Part model, mm, in its own coordinate system. A direction names the side the tool comes from. Round coordinates to 2 decimals unless told otherwise and drop trailing zeros. Loops run counter-clockwise (first coordinate to the right, second up) from the corner with the lowest first, then second, coordinate; pieces in that order, holes last.
(1) Mould opens along X. For faces 3 (the face through (516.086, -927, 1)), 4 (the face through (50, -1078, 1)), 5 (the face through (491, -1112.521, 1)) say: +X half, -X half, draft (parallel to the pull), parting line (faces both ways), or undercut.
(2) Flat gauge pins, fed straight in: pin 1 (5 mm diameter, centred on x = 457, z = 23, fed in from +Y); pin 2 (12 mm diameter, centred on x = 86.5, z = -0.5, fed in from +Y); pin 3 (2 mm diameter, centred on x = 250.5, z = 10, fed in from -Y). Where does each tip first touch, or does it go through?
(3) Cut at B-B on x = 88. List the corners of the cut face in (y, z), then the cut area to 3 significant figures.
(4) Cut at A-A on z = 4. List the corners of the cut face in (x, y), then the cut area to 3 significant figures.
(5) Tool access for faces 1 (the face through (255, -1042.521, 1)), 2 (the face through (0, -922, 1)): list every direction of +Z, -Z, +X, -X, +Y, -Y with a clear straight run to the whole face (end or side of a thin tool).
(6) Cut at C-C on y = -682.5. List the corners of the cut face in (x, z), then the cut area to 3 significant figures.
(7) Probe probe 1 along Y at (x, z) = (235.5, -16.5); probe 2 along Y at (x, z) = (193, -9); probe 3 along X at (y, z) = (-661.5, -22.5). List the from-to ranges inside material, lowest first.
from build123d import *

# Parameters (mm, degrees)
SKETCH_3_W      = 143.043199666
SKETCH_3_H      = 233.991238821
SKETCH_3_W_2    = 65
SKETCH_3_W_3    = 50
SKETCH_3_H_2    = 70
SKETCH_3_H_3    = 233.99123882
EXTRUDE_1_DEPTH = 45


with BuildPart() as part:
    # 草图3 → 凸台-拉伸1 (new, symmetric)
    with BuildSketch(Plane.XY):
        with Locations((394.564799499, -925.525377252)):
            Rectangle(SKETCH_3_W, SKETCH_3_H)
        with Locations((290.543199666, -925.525377252)):
            Rectangle(SKETCH_3_W_2, SKETCH_3_H)
        with Locations((225.543199666, -925.525377252)):
            Rectangle(SKETCH_3_W_2, SKETCH_3_H)
        with Locations((121.521599833, -925.525377252)):
            Rectangle(SKETCH_3_W, SKETCH_3_H)
        with Locations((25, -925.525377252)):
            Rectangle(SKETCH_3_W_3, SKETCH_3_H)
        with Locations((25, -1077.520996662)):
            Rectangle(SKETCH_3_W_3, SKETCH_3_H_2)
        with Locations((491.086399332, -1077.520996662)):
            Rectangle(SKETCH_3_W_3, SKETCH_3_H_2)
        with Locations((491.086399332, -925.525377252)):
            Rectangle(SKETCH_3_W_3, SKETCH_3_H)
        Polygon((466.086399332, -694.566015103), (466.086399332, -808.529757841), (516.086399332, -808.529757841), (516.086399332, -736.520996662), align=None)
        Polygon((323.043199666, -574.538519021), (323.043199666, -808.529757841), (466.086399332, -808.529757841), (466.086399332, -694.566015103), align=None)
        with Locations((290.543199666, -691.534138431)):
            Rectangle(SKETCH_3_W_2, SKETCH_3_H_3)
        with Locations((225.543199666, -691.534138431)):
            Rectangle(SKETCH_3_W_2, SKETCH_3_H_3)
        Polygon((50, -694.566015103), (50, -808.529757841), (193.043199666, -808.529757841), (193.043199666, -574.538519021), align=None)
        Polygon((0, -736.520996662), (0, -808.529757841), (50, -808.529757841), (50, -694.566015103), align=None)
    extrude(amount=EXTRUDE_1_DEPTH, both=True)


solid = part.part
Final values:
1. face 3: +X half
1. face 4: undercut
1. face 5: draft
2. pin 1: stops at y = -684.84
2. pin 2: stops at y = -658.9
2. pin 3: stops at y = -1042.52
3. outline: (-1042.52, -45) - (-662.68, -45) - (-662.68, 45) - (-1042.52, 45) - close
3. area: 34,200 mm2
4. outline: (0, -1112.52) - (50, -1112.52) - (50, -1042.52) - (466.09, -1042.52) - (466.09, -1112.52) - (516.09, -1112.52) - (516.09, -736.52) - (323.04, -574.54) - (193.04, -574.54) - (0, -736.52) - close
4. area: 217,000 mm2
5. face 1: +Z, -Z, -Y
5. face 2: +Z, -Z, -X, +Y, -Y
6. outline: (64.38, -45) - (451.71, -45) - (451.71, 45) - (64.38, 45) - close
6. area: 34,900 mm2
7. probe 1: y = -1042.52 to -574.54
7. probe 2: y = -1042.52 to -574.57
7. probe 3: x = 89.41 to 426.68
